Autodesk Fusion 360 part; units mm, degrees
sketch "スケッチ1" plane through (0, 0, 0) normal (0, 0, 1) x (1, 0, 0)
  line L0 (-9.5, 140) -> (-80.5, 140)
  line L1 (-80.5, 140) -> (-80.5, -140)
  line L2 (-80.5, -140) -> (-9.5, -140)
  line L3 (80.5, -130) -> (80.5, 130)
  line L4 (74.75, 130) -> (-80.5, -140) construction
  line L5 (-80.5, 140) -> (74.75, -130) construction
  line L6 (-9.5, 140) -> (-9.5, 130)
  line L7 (-9.5, 130) -> (80.5, 130)
  line L8 (-9.5, -140) -> (-9.5, -130)
  line L9 (-9.5, -130) -> (80.5, -130)
  dimension "d2" = 280
extrude "押し出し1" add sketch "スケッチ1" along normal blind 8
chamfer "面取り1" distance 25 angle 45 2 edges at (-80.5, -140, 4) (-80.5, 140, 4)
sketch "スケッチ2" plane through (0, 0, 8) normal (0, 0, 1) x (-1, 0, 0)
  line L0 (55.5, -140) -> (80.5, -115)
  line L1 (80.5, -115) -> (80.5, 115)
  line L2 (80.5, 115) -> (55.5, 140)
  line L3 (55.5, 140) -> (9.5, 140)
  line L4 (9.5, 140) -> (9.5, 130)
  line L5 (9.5, 130) -> (-80.5, 130)
  line L6 (-80.5, 130) -> (-80.5, -130)
  line L7 (-80.5, -130) -> (9.5, -130)
  line L8 (9.5, -130) -> (9.5, -140)
  line L9 (9.5, -140) -> (55.5, -140)
  line L10 (-80.5, -130) -> (-40.5, -130) construction
  line L11 (-40.5, -130) -> (-40.5, -70) construction
  line L12 (-40.5, -70) -> (-80.5, -70) construction
  line L13 (-80.5, -70) -> (-80.5, -130) construction
  line L14 (-40.5, -70) -> (-40.5, 0) construction
  line L15 (-40.5, 0) -> (-40.5, 70) construction
  point P0 (-40.5, -70)
  point P1 (-40.5, 0)
  point P2 (-40.5, 70)
  dimension "d10" = 40
  dimension "d11" = 60
  dimension "d12" = 70
  dimension "d13" = 70
hole "穴1" at (40.5, 70, 8) at (40.5, 0, 8) at (40.5, -70, 8) direction (0, 0, -1) diameter 22 end through all
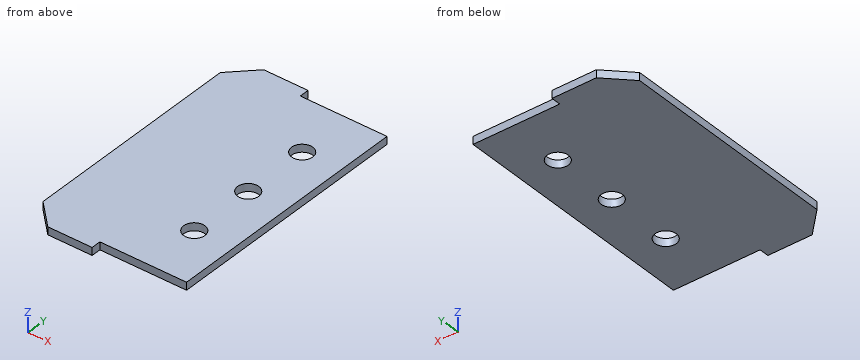
Model file for the job. Use its own axes, mm. Round coordinates to 2 decimals unless told otherwise and drop trailing zeros. Order: outer loops, then holes, each group sorted by start corner. A loop starts at its lowest first (then second) coordinate and runs counter-clockwise, first axis right, second up.
(1) Band-saw the part on A-A (y = -70). List the corners of the cut face in (x, z).
(2) Drill centre lines: line 1 (Y direction, x = 40.5, z = 3.25); line 2 (X direction, y = -70, z = 4.5); line 3 (X direction, y = 80, z = 1.5). Where is each one in solid material? Low to high.
(3) Band-saw the part on B-B (x = 40.5). List the corners of the cut face in (y, z), then the cut area to 3 significant figures.
(4) Pin check, flat tips, straight feed: pin 1 (2.5 mm diameter, centred on y = 135, z = 2.5, fed in from +X); pin 2 (4 mm diameter, centred on x = 51.5, z = 5, fed in from +Y); pin 3 (4 mm diameter, centred on x = 50, z = 2.5, fed in from -Y). Stop position of each tip, or through.
(5) Band-saw the part on D-D (y = -3). List the corners of the cut face in (x, z), then the cut area to 3 significant figures.
(6) Band-saw the part on C-C (z = 2). List the corners of the cut face in (x, y).
Verdict:
1. outline: (-80.5, 0) - (29.5, 0) - (29.5, 8) - (-80.5, 8) - close; (51.5, 0) - (80.5, 0) - (80.5, 8) - (51.5, 8) - close
2. line 1: y = -130 to -81, -59 to -11, 11 to 59, 81 to 130
2. line 2: x = -80.5 to 29.5, 51.5 to 80.5
2. line 3: x = -80.5 to 35.92, 45.08 to 80.5
3. outline: (-130, 0) - (-81, 0) - (-81, 8) - (-130, 8) - close; (-59, 0) - (-11, 0) - (-11, 8) - (-59, 8) - close; (11, 0) - (59, 0) - (59, 8) - (11, 8) - close; (81, 0) - (130, 0) - (130, 8) - (81, 8) - close
3. area: 1,550 mm2
4. pin 1: stops at x = -9.5
4. pin 2: stops at y = 130
4. pin 3: stops at y = -130
5. outline: (-80.5, 0) - (29.92, 0) - (29.92, 8) - (-80.5, 8) - close; (51.08, 0) - (80.5, 0) - (80.5, 8) - (51.08, 8) - close
5. area: 1,120 mm2
6. outline: (-80.5, -115) - (-55.5, -140) - (-9.5, -140) - (-9.5, -130) - (80.5, -130) - (80.5, 130) - (-9.5, 130) - (-9.5, 140) - (-55.5, 140) - (-80.5, 115) - close; hole circle Ø22 at (40.5, -70); hole circle Ø22 at (40.5, 0); hole circle Ø22 at (40.5, 70)
